Design review of the part built by this model. Coordinates are the model's own, in mm. A direction names the side the tool comes from. Give positions to 0.01 mm unless a question says otherwise; leave off trailing zeros. Loops run counter-clockwise (first coordinate to the right, second up) from the corner with the lowest first, then second, coordinate; pieces in that order, holes last. Notation, with made-up numbers: M -31,33 L -20,33 A29 ccw -20,59 Z; hole C 57.25,16 d8. An arc over 180 degrees is marked long. Use CSV: the item, a comma, the result in double quotes.
from build123d import *

# Parameters (mm, degrees)
BRIDA_BASE1_DEPTH                = 9.525
TALADRO_DE_MARGEN_PARA_M65_D     = 6.6
TALADRO_DE_MARGEN_PARA_M65_DEPTH = 11.62
TALADRO_DE_MARGEN_PARA_M65_TIP   = 1.982840043


# Sheet-metal steps are written as plain solids
with BuildPart() as part:
    # Croquis1 → Brida base1 (new, symmetric)
    with BuildSketch(Plane.XY):
        with BuildLine():
            Line((20, 11), (1, 11))
            ThreePointArc((1, 11), (0.292893219, 10.707106781), (0, 10))
            Line((0, 10), (0, 3))
            ThreePointArc((0, 3), (-0.878679656, 0.878679656), (-3, 0))
            Line((-3, 0), (-20, 0))
            Line((-20, 0), (-20, 2))
            Line((-20, 2), (-3, 2))
            ThreePointArc((-3, 2), (-2.292893219, 2.292893219), (-2, 3))
            Line((-2, 3), (-2, 10))
            ThreePointArc((-2, 10), (-1.121320344, 12.121320344), (1, 13))
            Line((1, 13), (20, 13))
            Line((20, 13), (20, 11))
        make_face()
    extrude(amount=BRIDA_BASE1_DEPTH, both=True)

    # Taladro de margen para M65
    with Locations(Plane(origin=(-10, 2, 0), x_dir=(1, 0, 0), z_dir=(0, 1, 0))):
        with Locations((0, 0)):
            Hole(TALADRO_DE_MARGEN_PARA_M65_D / 2, depth=TALADRO_DE_MARGEN_PARA_M65_DEPTH)
            with Locations((0, 0, -(TALADRO_DE_MARGEN_PARA_M65_DEPTH + TALADRO_DE_MARGEN_PARA_M65_TIP / 2))):  # 118° drill point
                Cone(0, TALADRO_DE_MARGEN_PARA_M65_D / 2, TALADRO_DE_MARGEN_PARA_M65_TIP, mode=Mode.SUBTRACT)


solid = part.part
(1) Machinability: for faces 5 (the flat face through (-14, 2, 0)), 6 (the flat face through (-13, 0, 2)), 7 (the flat face through (11, 11, 0)), which of the approach directions +Z, -Z, +X, -X, +Y, -Y give a long, thin tool a straight path to every point of the face, cutting with its end or side? Answer none if there is none.
A:
face 5,"+Z, -Z, -X, +Y"
face 6,"+Z, -Z, +X, -X, -Y"
face 7,"+Z, -Z, +X, -Y"
(2) We need section B-B on x = -10. State the section outline as (y, z) points (3 decimals), then the cut area to 3 significant figures.
A:
outline,"M 0,-9.525 L 2,-9.525 L 2,-3.3 L 0,-3.3 Z; M 0,3.3 L 2,3.3 L 2,9.525 L 0,9.525 Z"
area,"24.9 mm²"
(3) Clearance check with flat-ended pins moving along their axes: P1, Ø8, axis at x = 4.5, z = -3.5, coming from the -Y side; P2, Ø2, axis at y = 1.5, z = 2.5, coming from the +X side; P3, Ø1.5, axis at y = 10, z = -0.5, coming from the +X side; P4, Ø6, axis at x = -2, z = -2, coming from the -Y side. State where each tip first meets the part, or that it passes through.
A:
P1,"y = 10.87"
P2,"x = -0.04"
P3,"x = 0.34"
P4,"y = 0"
(4) The part is to be moulded in two halves that separate along X. For faces 1 (the cylindrical face through (-0.86, 0.9, 0.13)), 2 (the flat face through (-20, 1, 0)), 3 (the cylindrical face through (-6.7, 1, -0.1)), 4 (the flat face through (-1, 7, 9.525)), say which applies: released by +X, released by -X, zero draft, split by the parting line, or undercut.
A:
face 1,"released by +X"
face 2,"released by -X"
face 3,"undercut"
face 4,"zero draft"
(5) Wall thickness on line 1 along Z through (x, y) = (-10, 0.9) (3 decimals); line 2 along Y through (x, z) = (-5, 1.5); line 3 along Y through (x, z) = (12.5, 1.5): over which ranges is each line inside the solid? List them lowest first. Write a range as [from, to].
A:
line 1,"[-9.525, -3.3], [3.3, 9.525]"
line 2,"[0, 2]"
line 3,"[11, 13]"
(6) We need section A-A on z = 0. State the section outline as (x, y) points, then the cut area to 3 significant figures.
A:
outline,"M -20,0 L -13.3,0 L -13.3,2 L -20,2 Z; M -6.7,0 L -3,0 A3 ccw 0,3 L 0,10 A1 cw 1,11 L 20,11 L 20,13 L 1,13 A3 ccw -2,10 L -2,3 A1 cw -3,2 L -6.7,2 Z"
area,"85.4 mm²"
(7) We need section D-D on x = 2. State the section outline as (y, z) points (3 decimals).
A:
outline,"M 11,-9.525 L 13,-9.525 L 13,9.525 L 11,9.525 Z"
(8) We need section C-C on z = 4.75. State the section outline as (x, y) points.
A:
outline,"M -20,0 L -3,0 A3 ccw 0,3 L 0,10 A1 cw 1,11 L 20,11 L 20,13 L 1,13 A3 ccw -2,10 L -2,3 A1 cw -3,2 L -20,2 Z"
